```python
from build123d import *

# Parameters (mm, degrees)
F0_W     = 19.75
F0_H     = 65
F0_W_2   = 7.2
F0_H_2   = 37
F1_DEPTH = 4.7
F2_DEPTH = 3.7
F4_DEPTH = 4.701


with BuildPart() as f1:
    # F0 (on Front) → F1 (new body)
    with BuildSketch(Plane.XZ):
        with Locations((9.875, 32.5)):
            Rectangle(F0_W, F0_H)
        with Locations((9.875, 20)):
            Rectangle(F0_W_2, F0_H_2, mode=Mode.SUBTRACT)
    extrude(amount=F1_DEPTH)

    # F0 (on Front) → F2 (join)
    with BuildSketch(Plane.XZ):
        with Locations((9.875, 20)):
            Rectangle(F0_W_2, F0_H_2)
    extrude(amount=F2_DEPTH)

    # F3 (on face) → F4 (cut, through all)
    with BuildSketch(Plane(origin=(0, 0, 0), x_dir=(-1, 0, 0), z_dir=(0, 1, 0))):
        with BuildLine():
            ThreePointArc((-19.75, 53.2128467794), (-18.6419559311, 55.3359042131), (-18.2596136294, 57.7))
            ThreePointArc((-18.2596136294, 57.7), (-18.6419559311, 60.0640957869), (-19.75, 62.1871532206))
            Line((-19.75, 62.1871532206), (-19.75, 53.2128467794))
        make_face()
        with BuildLine():
            Line((0, 53.2128467794), (0, 62.1871532206))
            ThreePointArc((0, 62.1871532206), (-1.4903863706, 57.7), (0, 53.2128467794))
        make_face()
    extrude(amount=-F4_DEPTH, mode=Mode.SUBTRACT)


solid = f1.part
```
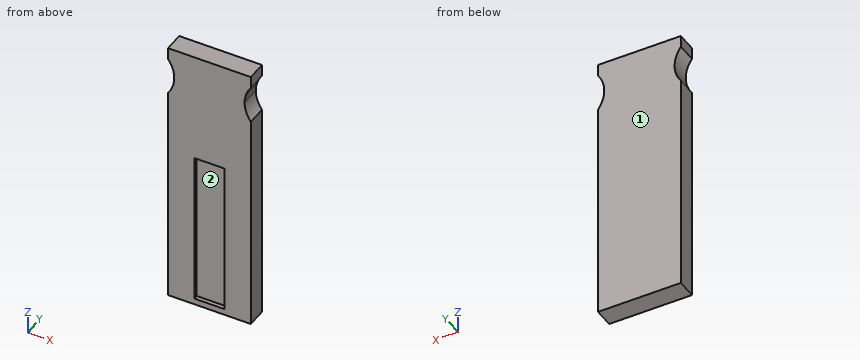
Could you check a few things on this model? Use its own coordinates, in mm. Face numbers are marked on the shaded views. Round coordinates to 2 decimals unless told otherwise and drop trailing zeros. Loops run counter-clockwise (first coordinate to the right, second up) from the corner with the lowest first, then second, coordinate; pieces in that order, holes last. Notation, with made-up numbers: M 60,25.5 L 87,25.5 A12 cw 87,47.5 Z; hole C -12.75,13 d11. An arc over 180 degrees is marked long. Answer as CSV lines item,"result".
1) We'd pull the mould along Z, two halves only. Please class the marked faces 1 and 2: released by +Z, released by -Z, zero draft, split by the parting line, or undercut.
From the geometry:
face 1,"zero draft"
face 2,"undercut"
2) Imagine slicing it at A-A on z = 20.5. List the corners of the cut face in (x, y) for me (3 decimals), and give its area (3 significant figures).
From the geometry:
outline,"M 0,-4.7 L 6.275,-4.7 L 6.275,-3.7 L 13.475,-3.7 L 13.475,-4.7 L 19.75,-4.7 L 19.75,0 L 0,0 Z"
area,"85.6 mm^2"
3) For pin 1 Ø6 at (x, z) = (9.5, 13) entering from -Y; pin 2 Ø1.5 at (y, z) = (-1, 58.5) entering from +X, each with a flat end and sliding along its axis, tell me the tip position at first contact or that it passes through.
From the geometry:
pin 1,"y = -3.7"
pin 2,"x = 18.42"
4) Imagine slicing it at B-B on x = 12.75. List the corners of the cut face in (y, z) for me, and give its area (4 significant figures).
From the geometry:
outline,"M -4.7,0 L 0,0 L 0,65 L -4.7,65 L -4.7,38.5 L -3.7,38.5 L -3.7,1.5 L -4.7,1.5 Z"
area,"268.5 mm^2"
5) Imagine slicing it at C-C on z = 54. List the corners of the cut face in (x, y) for me.
From the geometry:
outline,"M 0.51,-4.7 L 19.24,-4.7 L 19.24,0 L 0.51,0 Z"
6) If I drill on probe 1 along X at (y, z) = (-4.2, 30.5) (3 decimals); probe 2 along Y at (x, z) = (9, 29); probe 3 along X at (y, z) = (-4.35, 57.5), over which ranges is the centre line in solid material (lowest first)?
From the geometry:
probe 1,"0 to 6.275, 13.475 to 19.75"
probe 2,"-3.7 to 0"
probe 3,"1.49 to 18.26"
